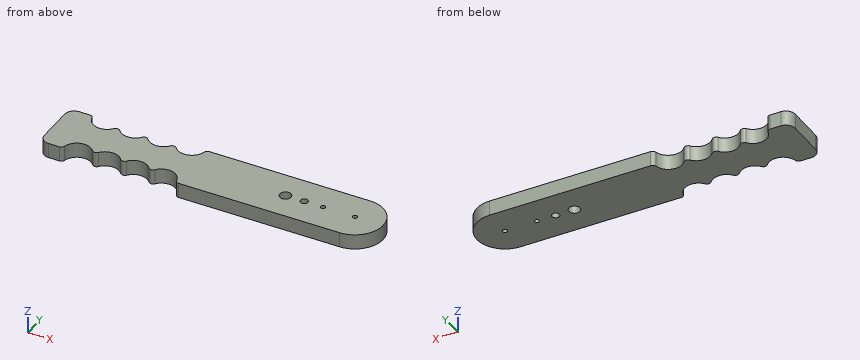
from build123d import *

# Parameters (mm, degrees)
SKETCH1_R           = 1.25
SKETCH1_R_2         = 3
SKETCH1_R_3         = 2
BOSS_EXTRUDE1_DEPTH = 8
FILLET1_R           = 5
FILLET2_R           = 2


with BuildPart() as part:
    # Sketch1 → Boss-Extrude1 (new body)
    with BuildSketch(Plane.XY):
        with BuildLine():
            Line((0, 15), (-87.5, 15))
            ThreePointArc((-87.5, 15), (-95, 7.5), (-102.5, 15))
            ThreePointArc((-102.5, 15), (-110, 7.5), (-117.5, 15))
            ThreePointArc((-117.5, 15), (-125, 7.5), (-132.5, 15))
            ThreePointArc((-132.5, 15), (-140, 7.5), (-147.5, 15))
            Line((-147.5, 15), (-160, 15))
            Line((-160, 15), (-160, -15))
            Line((-160, -15), (-147.5, -15))
            ThreePointArc((-147.5, -15), (-140, -7.5), (-132.5, -15))
            ThreePointArc((-132.5, -15), (-125, -7.5), (-117.5, -15))
            ThreePointArc((-117.5, -15), (-110, -7.5), (-102.5, -15))
            ThreePointArc((-102.5, -15), (-95, -7.5), (-87.5, -15))
            Line((-87.5, -15), (0, -15))
            ThreePointArc((0, -15), (15, 0), (0, 15))
        make_face()
        Circle(SKETCH1_R, mode=Mode.SUBTRACT)
        with Locations((-17, 0)):
            Circle(SKETCH1_R, mode=Mode.SUBTRACT)
        with Locations((-37, 0)):
            Circle(SKETCH1_R_2, mode=Mode.SUBTRACT)
        with Locations((-27, 0)):
            Circle(SKETCH1_R_3, mode=Mode.SUBTRACT)
    extrude(amount=BOSS_EXTRUDE1_DEPTH)

    # Fillet1
    fillet1_edges = [part.edges().sort_by_distance(p)[0] for p in [
        (-160, -15, 4),
        (-160, 15, 4),
    ]]
    fillet(fillet1_edges, radius=FILLET1_R)

    # Fillet2
    fillet2_edges = [part.edges().sort_by_distance(p)[0] for p in [
        (-87.5, -15, 4),
        (-102.5, -15, 4),
        (-117.5, -15, 4),
        (-132.5, -15, 4),
        (-147.5, -15, 4),
        (-147.5, 15, 4),
        (-132.5, 15, 4),
        (-117.5, 15, 4),
        (-102.5, 15, 4),
        (-87.5, 15, 4),
    ]]
    fillet(fillet2_edges, radius=FILLET2_R)


solid = part.part
Input: part model. Units: mm. Frame: model coordinates. Give positions to 0.01 mm unless a question says otherwise; leave off trailing zeros. Write each loop counter-clockwise with the first axis right and the second up, starting at its lowest first coordinate (ties: lowest second). Pieces come first, ordered by that corner, then holes. Notation, with made-up numbers: (66, 13) -> (88, 13) arc R23 cw to (88, 51) -> close; hole circle Ø7 at (21.5, -17.5). An arc over 180 degrees is marked (long way). Use one line per item in the form item = value. Start each with the question number.
1) Section query C-C on x = -93. Return the cut outline in (y, z).
2) Pin query (flat end, axial travel): pin 1 (2 mm diameter, centred on x = -17, y = 0, fed in from +Z); pin 2 (1 mm diameter, centred on y = 11.5, z = 2.5, fed in from -X); pin 3 (3 mm diameter, centred on y = -5, z = 4.5, fed in from +X). Return the tip coordinate at first contact, or that it passes through.
3) Ray query, probe 1 along X at (y, z) = (1.5, 3.75); probe 2 along X at (y, z) = (10, 1.25); probe 3 along X at (y, z) = (-11, 2.5). Return the intervals inside material, ascending. Write a range as from..to.
4) Section query A-A on x = -37. Return the cut outline in (y, z), then the cut area to 3 significant figures.
5) Section query D-D on x = 4. Return the cut outline in (y, z).
6) Section query B-B on z = 4.5. Count the separate pieces of the cut face and the enclosed holes in it, then the cut area to 3 significant figures.
Outcome:
q1.outline = (-7.77, 0) -> (7.77, 0) -> (7.77, 8) -> (-7.77, 8) -> close
q2.pin_1 = through
q2.pin_2 = -159.9
q2.pin_3 = 14.59
q3.probe_1 = -160..-39.6, -34.4..-28.32, -25.68..14.92
q3.probe_2 = -160..-145.59, -134.41..-130.59, -119.41..-115.59, -104.41..-100.59, -89.41..11.18
q3.probe_3 = -159.9..-146.34, -133.3..-131.7, -118.3..-116.7, -103.3..-101.7, -88.66..10.2
q4.outline = (-15, 0) -> (-3, 0) -> (-3, 8) -> (-15, 8) -> close; (3, 0) -> (15, 0) -> (15, 8) -> (3, 8) -> close
q4.area = 192 mm^2
q5.outline = (-14.46, 0) -> (14.46, 0) -> (14.46, 8) -> (-14.46, 8) -> close
q6.separate_pieces = 1
q6.enclosed_holes = 4
q6.area = 4,370 mm^2
